Can you work these out from the model? Positions are in its coordinate system, mm. A direction names the side the tool comes from. Round coordinates to 2 decimals unless told otherwise and drop trailing zeros. Write each loop counter-clockwise with the first axis right and the second up, starting at its lowest first coordinate (ties: lowest second). Pieces come first, ordered by that corner, then holes. Notation, with made-up numbers: M 74.5,2.25 L 132.5,2.25 A14 cw 132.5,19.25 Z; hole C -8.5,15 d1. An arc over 180 degrees is marked long. Answer in a Markdown table with one row per item. Add a question column.
(1) Suppose I cut it at A-A, the plane y = 0. Write out the boundary of the cut face in (x, z).
(2) Suppose I cut it at C-C, the plane z = 26. Write out the boundary of the cut face in (x, y).
(3) If I drill on probe 1 along Y at (x, z) = (0.5, 107.5); probe 2 along Y at (x, z) = (-8.75, 81.5); probe 3 along X at (y, z) = (2, 49.5), over which ranges is the centre line in solid material (lowest first)?
(4) Suppose I cut it at D-D, the plane y = -7.25. Write out the boundary of the cut face in (x, z), then the cut area to 3 significant figures.
(5) For faces 1 (the face through (9.933, 3.128, 94.094)), 2 (the face through (-1.82, 1.67, 6.26)), which set-ups out of +Z, -Z, +X, -X, +Y, -Y let a thin tool reach every point of the face, with its end or its side?
(6) I'm going to push flat-ended pins straight in: pin 1 (1 mm diameter, centred on x = 4.5, y = -8.5, fed in from -Z); pin 2 (8 mm diameter, centred on x = -0.5, y = -5.5, fed in from +Z); pin 3 (12 mm diameter, centred on x = 7.5, z = 66.5, fed in from +Y); pin 4 (3 mm diameter, centred on y = -6.5, z = 49, fed in from -X). Where does each tip first touch, or does it pass through?
(7) If we mould it in two halves opening along Y, with no side actions, what happens to faces 3 (the face through (2, -2, 12.7)), 4 (the face through (-2.671, -12.026, 87.655)), 5 (the face through (3, 0, 0))? For each: released by +Y, released by -Y, zero draft, split by the parting line, or undercut.
from build123d import *

# Parameters (mm, degrees)
F0_R     = 12.319
F0_R_2   = 10.414
F1_DEPTH = 177.8
F0_R_3   = 2.471855
F2_DEPTH = 12.7
F3_DEPTH = 25.4


with BuildPart() as f1:
    # F0 (on Top) → F1 (new body)
    with BuildSketch(Plane.XY):
        Circle(F0_R)
        Circle(F0_R_2, mode=Mode.SUBTRACT)
    extrude(amount=F1_DEPTH)

    # F0 (on Top) → F2 (join)
    with BuildSketch(Plane.XY):
        Circle(F0_R_2)
        Circle(F0_R_3, mode=Mode.SUBTRACT)
    extrude(amount=F2_DEPTH)

    # F0 (on Top) → F3 (cut)
    with BuildSketch(Plane.XY):
        Circle(F0_R_3)
    extrude(amount=-F3_DEPTH, mode=Mode.SUBTRACT)


solid = f1.part
Calculated:
| question | item | result |
|---|---|---|
| 1 | outline | M -12.32,0 L -2.47,0 L -2.47,12.7 L -10.41,12.7 L -10.41,177.8 L -12.32,177.8 Z; M 2.47,0 L 12.32,0 L 12.32,177.8 L 10.41,177.8 L 10.41,12.7 L 2.47,12.7 Z |
| 2 | outline | C 0,0 d24.64; hole C 0,0 d20.83 |
| 3 | probe 1 | -12.31 to -10.4, 10.4 to 12.31 |
| 3 | probe 2 | -8.67 to -5.65, 5.65 to 8.67 |
| 3 | probe 3 | -12.16 to -10.22, 10.22 to 12.16 |
| 4 | outline | M -9.96,0 L 9.96,0 L 9.96,177.8 L 7.48,177.8 L 7.48,12.7 L -7.48,12.7 L -7.48,177.8 L -9.96,177.8 Z |
| 4 | area | 1,070 mm² |
| 5 | face 1 | +Z |
| 5 | face 2 | +Z, -Z |
| 6 | pin 1 | z = 0 |
| 6 | pin 2 | z = 12.7 |
| 6 | pin 3 | y = 12.23 |
| 6 | pin 4 | x = -11.26 |
| 7 | face 3 | undercut |
| 7 | face 4 | split by the parting line |
| 7 | face 5 | zero draft |
